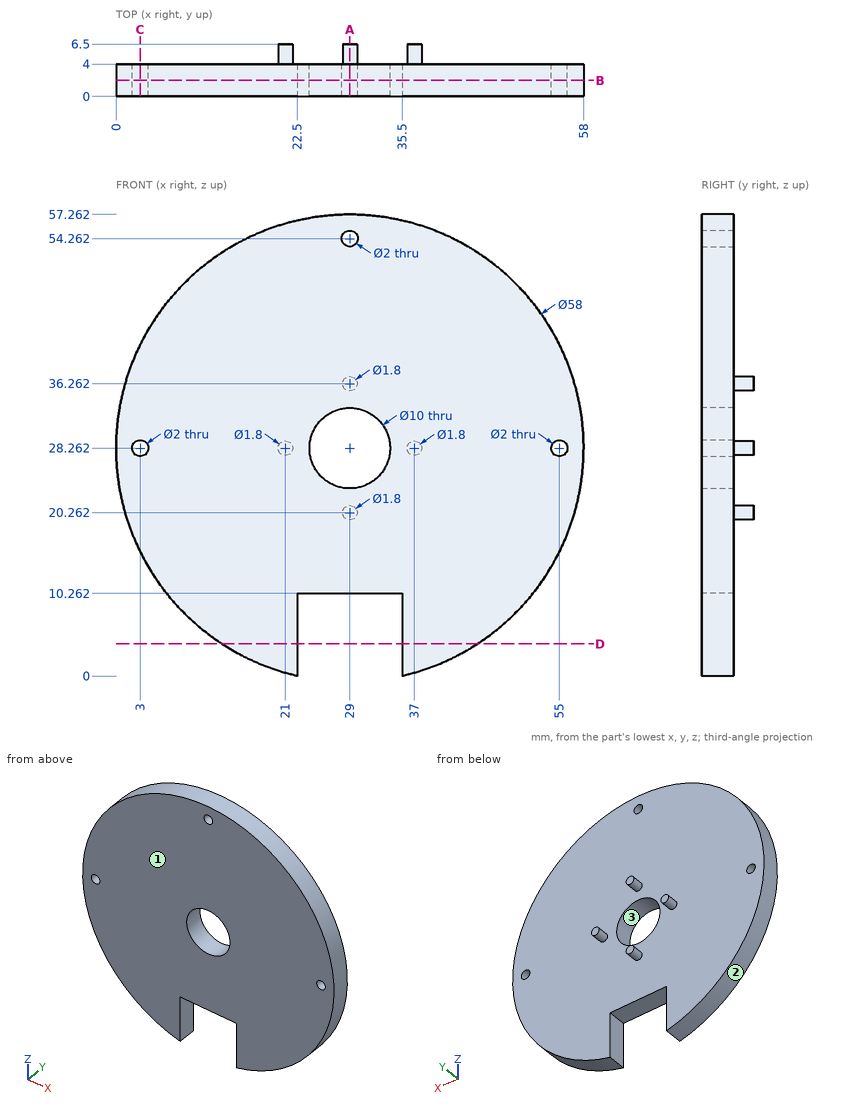
The drawing under review shows one solid part. Ordinate dimensions are in mm from its lowest x, y, z. Round coordinates to 2 decimals unless told otherwise and drop trailing zeros. Loops run counter-clockwise (first coordinate to the right, second up) from the corner with the lowest first, then second, coordinate; pieces in that order, holes last. Notation, with made-up numbers: M 48.25,54 L 91.25,54 A13 cw 91.25,60 Z; hole C 88.25,-35.5 d8. An arc over 180 degrees is marked long. Answer as CSV lines item,"result". Start each with the question number.
Item 1: Consider section A-A (x = 29). Write out the cut boundary in (y, z), then the cut area to 3 significant figures.
Item 2: Mouldability with a two-part tool opening along X and no side actions: class the marked faces 1, 2 and 3 as released by +X, released by -X, zero draft, split by the parting line, or undercut.
Item 3: Consider section C-C (x = 3). Write out the cut boundary in (y, z).
Item 4: Wall thickness on line 1 (Y direction, x = 10.5, z = 36); line 2 (X direction, y = 3.5, z = 27.5); line 3 (Z direction, x = 25.5, y = 2): over which ranges is each line inside the solid? List them lowest first. Write a range as [from, to].
Item 5: Insertion check: P1, Ø3, axis at y = 3, z = 3, coming from the -X side; P2, Ø3, axis at x = 32, y = 2.5, coming from the -Z side; P3, Ø1, axis at x = 17.5, y = 1.5, coming from the +Z side (3 decimals). Each pin has a flat end and moves straight along its axis. Give the tip position at first contact, or say it passes through.
Item 6: Consider section B-B (y = 2). Write out the cut boundary in (x, z).
Item 7: Consider section D-D (z = 4). Write out the cut boundary in (x, y), then the cut area to 3 significant figures.
Answer:
1,outline,"M 0,10.26 L 4,10.26 L 4,19.36 L 6.5,19.36 L 6.5,21.16 L 4,21.16 L 4,23.26 L 0,23.26 Z; M 0,33.26 L 4,33.26 L 4,35.36 L 6.5,35.36 L 6.5,37.16 L 4,37.16 L 4,53.26 L 0,53.26 Z; M 0,55.26 L 4,55.26 L 4,57.26 L 0,57.26 Z"
1,area,"149 mm^2"
2,face 1,"zero draft"
2,face 2,"split by the parting line"
2,face 3,"undercut"
3,outline,"M 0,15.42 L 4,15.42 L 4,27.26 L 0,27.26 Z; M 0,29.26 L 4,29.26 L 4,41.11 L 0,41.11 Z"
4,line 1,"y = [0, 4]"
4,line 2,"x = [0.01, 2.35], [3.65, 24.06], [33.94, 54.35], [55.65, 57.99]"
4,line 3,"z = [10.26, 24.69], [31.83, 57.05]"
5,P1,"stops at x = 12.38"
5,P2,"stops at z = 10.26"
5,P3,"stops at z = 55.095"
6,outline,"M 22.5,0 L 22.5,10.26 L 35.5,10.26 L 35.5,0 A29 ccw long Z; hole C 3,28.26 d2; hole C 29,28.26 d10; hole C 29,54.26 d2; hole C 55,28.26 d2"
7,outline,"M 13.11,0 L 22.5,0 L 22.5,4 L 13.11,4 Z; M 35.5,0 L 44.89,0 L 44.89,4 L 35.5,4 Z"
7,area,"75.1 mm^2"
